```python
from build123d import *

# Parameters (mm, degrees)
SKETCH_1_W               = 40
SKETCH_1_H               = 20
EXTRUDE_1_DEPTH          = 40
CUT_EXTRUDE_1_DEPTH      = 49.989794856
CUT_EXTRUDE_1_DEPTH_BACK = 49.989794856
SKETCH_4_R               = 4
CUT_EXTRUDE_3_DEPTH      = 46.82575695
SKETCH_5_R               = 5
SKETCH_5_R_2             = 2
EXTRUDE_2_DEPTH          = 4


with BuildPart() as part:
    # 草图1 → 凸台-拉伸1 (new body)
    with BuildSketch(Plane(origin=(0, 0, 0), x_dir=(1, 0, 0), z_dir=(0, 1, 0))):
        Rectangle(SKETCH_1_W, SKETCH_1_H)
    extrude(amount=EXTRUDE_1_DEPTH)

    # 草图2 → 切除-拉伸1 (cut, two sides: drawn at the far end of the back side and taken through both)
    with BuildSketch(Plane.XY.offset(10).offset(-CUT_EXTRUDE_1_DEPTH_BACK)):
        Polygon((-15, 156.301458127), (-15, 40), (-15, 4), (15, 4), (15, 40), (15, 156.301458127), (15, 388.904374382), (-15, 388.904374382), align=None)
    extrude(amount=CUT_EXTRUDE_1_DEPTH + CUT_EXTRUDE_1_DEPTH_BACK, mode=Mode.SUBTRACT)

    # 草图4 → 切除-拉伸3 (cut, through all)
    with BuildSketch(Plane.XZ):
        with Locations(Location((0, 0, 0), (0, 0, 270))):
            Circle(SKETCH_4_R)
    extrude(amount=-CUT_EXTRUDE_3_DEPTH, mode=Mode.SUBTRACT)

    # 草图5 → 凸台-拉伸2 (add)
    with BuildSketch(Plane(origin=(-15, 0, 0), x_dir=(0, 0, -1), z_dir=(1, 0, 0))):
        with Locations(Location((0, 30, 0), (0, 0, 90))):
            Circle(SKETCH_5_R)
        with Locations(Location((0, 30, 0), (0, 0, 90))):
            Circle(SKETCH_5_R_2, mode=Mode.SUBTRACT)
    extrude_2 = extrude(amount=EXTRUDE_2_DEPTH)

    # 镜向1: 凸台-拉伸2 across plane
    add(extrude_2.mirror(Plane(origin=(0, 0, 0), x_dir=(0, 0, 1), z_dir=(1, 0, 0))))


solid = part.part
```
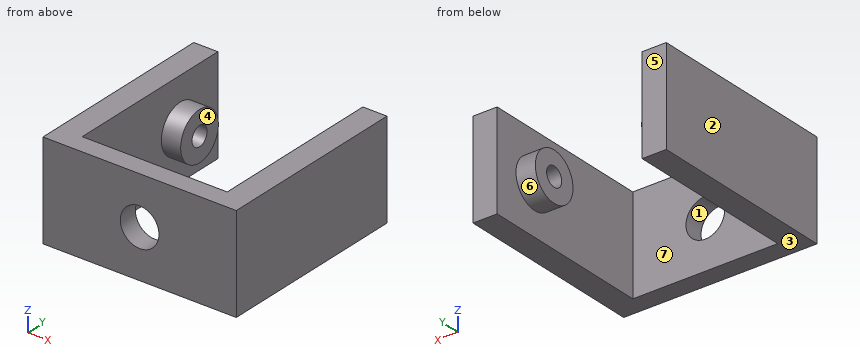
Check sheet for the modelled part. Datum: model origin and axes. Units: mm. Face numbers are marked on the shaded views. A direction names the side the tool comes from. Round coordinates to 2 decimals unless told otherwise and drop trailing zeros. Order: outer loops, then holes, each group sorted by start corner. A loop starts at its lowest first (then second) coordinate and runs counter-clockwise, first axis right, second up. Notation, with made-up numbers: (30.5, 9.5) -> (60.5, 9.5) arc R25 ccw to (60.5, 24.5) -> close; hole circle Ø6 at (-23, 30.25). An arc over 180 degrees is marked (long way). Use CSV: the item, a comma, the result in double quotes.
(1) Material ranges on line 1 along X through (y, z) = (5.5, 9); line 2 along X through (y, z) = (32, -3.25); line 3 along Z through (x, y) = (13.45, 30), recorded low to high. Write a range as from..to.
Worked out:
line 1,"-20..-15, 15..20"
line 2,"-20..-11, 11..20"
line 3,"-5..-2, 2..5"
(2) Depth check by flat-ended pin: pin 1 (6 mm diameter, centred on x = -7.5, z = 6.5, fed in from +Y). Enter the tip coordinate at first touch or a pass-through.
Worked out:
pin 1,"y = 4"
(3) Draft check along X on the marked faces 1, 2 and 3. Enter one of: pulls with the +X half, pulls with the -X half, needs draft (parallel to the pull), parting line crosses it, or undercut.
Worked out:
face 1,"undercut"
face 2,"pulls with the -X half"
face 3,"needs draft"
(4) Cross-section at D-D (x = 0). Record the boundary of the cut face in (y, z), and give its area (3 significant figures).
Worked out:
outline,"(0, -10) -> (4, -10) -> (4, -4) -> (0, -4) -> close; (0, 4) -> (4, 4) -> (4, 10) -> (0, 10) -> close"
area,"48.0 mm²"
(5) Cross-section at C-C (y = 30). Record the boundary of the cut face in (x, z), and give its area (3 significant figures).
Worked out:
outline,"(-20, -10) -> (-15, -10) -> (-15, -5) -> (-11, -5) -> (-11, -2) -> (-15, -2) -> (-15, 2) -> (-11, 2) -> (-11, 5) -> (-15, 5) -> (-15, 10) -> (-20, 10) -> close; (11, -5) -> (15, -5) -> (15, -10) -> (20, -10) -> (20, 10) -> (15, 10) -> (15, 5) -> (11, 5) -> (11, 2) -> (15, 2) -> (15, -2) -> (11, -2) -> close"
area,"248 mm²"
(6) Cross-section at B-B (z = 0). Record the boundary of the cut face in (x, y), and give its area (3 significant figures).
Worked out:
outline,"(-20, 0) -> (-4, 0) -> (-4, 4) -> (-15, 4) -> (-15, 25) -> (-11, 25) -> (-11, 28) -> (-15, 28) -> (-15, 32) -> (-11, 32) -> (-11, 35) -> (-15, 35) -> (-15, 40) -> (-20, 40) -> close; (4, 0) -> (20, 0) -> (20, 40) -> (15, 40) -> (15, 35) -> (11, 35) -> (11, 32) -> (15, 32) -> (15, 28) -> (11, 28) -> (11, 25) -> (15, 25) -> (15, 4) -> (4, 4) -> close"
area,"536 mm²"
(7) Tool access check on the marked faces 4, 5, 6 and 7. Record the directions out of +Z, -Z, +X, -X, +Y, -Y that give a thin tool (end or side, any length) a straight path to the whole face; none if there is none.
Worked out:
face 4,"+Z, -Z, +Y"
face 5,"+Z, -Z, +X, -X, +Y"
face 6,"none"
face 7,"+Z, -Z"
(8) Cross-section at A-A (x = -12). Record the boundary of the cut face in (y, z).
Worked out:
outline,"(0, -10) -> (4, -10) -> (4, 10) -> (0, 10) -> close; circle Ø10 at (30, 0); hole circle Ø4 at (30, 0)"
